from build123d import *

# Parameters (mm, degrees)
SKETCH_1_W          = 40
SKETCH_1_H          = 150
EXTRUDE_1_DEPTH     = 6
SKETCH_3_W          = 30
SKETCH_3_H          = 59
SKETCH_3_H_2        = 58
CUT_EXTRUDE_2_DEPTH = 156.357651888
SKETCH_4_W          = 35
SKETCH_4_H          = 64
SKETCH_4_H_2        = 63
CUT_EXTRUDE_3_DEPTH = 3.5
FILLET_2_R          = 5
SKETCH_7_W          = 40
SKETCH_7_H          = 9.998672315
EXTRUDE_2_DEPTH     = 4
SKETCH_5_W          = 40
SKETCH_5_H          = 8.05
CUT_EXTRUDE_4_DEPTH = 2
SKETCH_8_R          = 2.4
CUT_EXTRUDE_5_DEPTH = 6
SKETCH_9_R          = 1.8
CUT_EXTRUDE_6_DEPTH = 156.357651888


with BuildPart() as part:
    # ｽｹｯﾁ1 → ﾎﾞｽ - 押し出し1 (new body)
    with BuildSketch(Plane.XY):
        with Locations((20, 75)):
            Rectangle(SKETCH_1_W, SKETCH_1_H)
    extrude(amount=EXTRUDE_1_DEPTH)

    # ｽｹｯﾁ3 → ｶｯﾄ - 押し出し2 (cut, through all)
    with BuildSketch(Plane.XY.offset(6)):
        with Locations((20, 108.5)):
            Rectangle(SKETCH_3_W, SKETCH_3_H)
        with Locations((20, 42)):
            Rectangle(SKETCH_3_W, SKETCH_3_H_2)
    extrude(amount=-CUT_EXTRUDE_2_DEPTH, mode=Mode.SUBTRACT)

    # ｽｹｯﾁ4 → ｶｯﾄ - 押し出し3 (cut)
    with BuildSketch(Plane.XY.offset(6)):
        with Locations((20, 108.5)):
            Rectangle(SKETCH_4_W, SKETCH_4_H)
        with Locations((20, 42)):
            Rectangle(SKETCH_4_W, SKETCH_4_H_2)
    extrude(amount=-CUT_EXTRUDE_3_DEPTH, mode=Mode.SUBTRACT)

    # ﾌｨﾚｯﾄ2
    fillet_2_edges = [part.edges().sort_by_distance(p)[0] for p in [
        (35, 138, 1.25),
        (35, 79, 1.25),
        (5, 79, 1.25),
        (5, 138, 1.25),
        (35, 71, 1.25),
        (35, 13, 1.25),
        (5, 13, 1.25),
        (5, 71, 1.25),
        (2.5, 76.5, 4.25),
        (2.5, 140.5, 4.25),
        (37.5, 140.5, 4.25),
        (37.5, 76.5, 4.25),
        (2.5, 10.5, 4.25),
        (2.5, 73.5, 4.25),
        (37.5, 73.5, 4.25),
        (37.5, 10.5, 4.25),
    ]]
    fillet(fillet_2_edges, radius=FILLET_2_R)

    # ｽｹｯﾁ7 → ﾎﾞｽ - 押し出し2 (add)
    with BuildSketch(Plane.XY.offset(6)):
        with Locations((20, 4.999336158)):
            Rectangle(SKETCH_7_W, SKETCH_7_H)
    extrude(amount=EXTRUDE_2_DEPTH)

    # ｽｹｯﾁ5 → ｶｯﾄ - 押し出し4 (cut)
    with BuildSketch(Plane.XY.offset(6)):
        with Locations((20, 145.975)):
            Rectangle(SKETCH_5_W, SKETCH_5_H)
    extrude(amount=-CUT_EXTRUDE_4_DEPTH, mode=Mode.SUBTRACT)

    # ｽｹｯﾁ8 → ｶｯﾄ - 押し出し5 (cut)
    with BuildSketch(Plane.XZ):
        with Locations(Location((5, 6, 0), (0, 0, 270))):
            Circle(SKETCH_8_R)
        with Locations(Location((25, 6, 0), (0, 0, 270))):
            Circle(SKETCH_8_R)
        with Locations(Location((35, 6, 0), (0, 0, 270))):
            Circle(SKETCH_8_R)
        with Locations(Location((15, 6, 0), (0, 0, 270))):
            Circle(SKETCH_8_R)
    extrude(amount=-CUT_EXTRUDE_5_DEPTH, mode=Mode.SUBTRACT)

    # ｽｹｯﾁ9 → ｶｯﾄ - 押し出し6 (cut, through all)
    with BuildSketch(Plane.XY.offset(4)):
        with Locations((4, 146)):
            Circle(SKETCH_9_R)
        with Locations((36, 146)):
            Circle(SKETCH_9_R)
    extrude(amount=-CUT_EXTRUDE_6_DEPTH, mode=Mode.SUBTRACT)


solid = part.part
The listing builds one solid part. Answer for the finished solid, in the listing's coordinates (mm). A direction names the side the tool comes from. Give positions to 0.01 mm unless a question says otherwise; leave off trailing zeros. Write each loop counter-clockwise with the first axis right and the second up, starting at its lowest first coordinate (ties: lowest second). Pieces come first, ordered by that corner, then holes.
1) Section B-B (x = 15) is taken. Write down the section's boundary in (y, z), and give its area (3 significant figures).
2) Section A-A (y = 53) is taken. Write down the section's boundary in (x, z).
3) For a pull along X with two mould halves and no side action, classify faces 1 (the face through (40, 74, 3)), 2 (the face through (35, 42, 1)), 3 (the face through (20, 76, 0)) as pulls with the +X half, pulls with the -X half, needs draft (parallel to the pull), parting line crosses it, or undercut.
4) Find the intervals of material crossed by L1, parallel to Y at x = 27, z = 1.25; L2, parallel to X at y = 4.1, z = 6; L3, parallel to Y at x = 29, z = 5.5, in increasing order.
5) Given P1, Ø1.4, axis at x = 26, z = 6.5, coming from the -Y side; P2, Ø4.5, axis at x = 27, z = 8, coming from the +Y side, each flat-ended and moving along its own axis, determine where each tip first touches the part or whether it passes through.
6) A tool of negligible diameter and unlimited length cuts with its end or side. For faces 4 (the face through (20, 76.5, 4)), 5 (the face through (32.657, 2.958, 6.52)), 6 (the face through (20, 71, 1)), from which of +Z, -Z, +X, -X, +Y, -Y can it reach the whole face along a straight path? Write none if from no direction.
Response:
1. outline: (0, 0) - (13, 0) - (13, 2.5) - (10.5, 2.5) - (10.5, 6) - (10, 6) - (10, 10) - (0, 10) - (0, 8.4) - (6, 8.4) - (6, 3.6) - (0, 3.6) - close; (71, 0) - (79, 0) - (79, 2.5) - (76.5, 2.5) - (76.5, 6) - (73.5, 6) - (73.5, 2.5) - (71, 2.5) - close; (138, 0) - (150, 0) - (150, 4) - (141.95, 4) - (141.95, 6) - (140.5, 6) - (140.5, 2.5) - (138, 2.5) - close
1. area: 158 mm2
2. outline: (0, 0) - (5, 0) - (5, 2.5) - (2.5, 2.5) - (2.5, 6) - (0, 6) - close; (35, 0) - (40, 0) - (40, 6) - (37.5, 6) - (37.5, 2.5) - (35, 2.5) - close
3. face 1: pulls with the +X half
3. face 2: undercut
3. face 3: needs draft
4. L1: y = 0 to 13, 71 to 79, 138 to 150
4. L2: x = 0 to 2.6, 7.4 to 12.6, 17.4 to 22.6, 27.4 to 32.6, 37.4 to 40
4. L3: y = 0 to 10.5, 73.5 to 76.5, 140.5 to 141.95
5. P1: stops at y = 6
5. P2: stops at y = 141.95
6. face 4: +Z
6. face 5: -Y
6. face 6: +Z, -Z
